Source: CAD feature listing. Evaluate the final solid. Frame: model axes, mm. A direction names the side the tool comes from. Give positions to 0.01 mm unless a question says otherwise; leave off trailing zeros. Order: outer loops, then holes, each group sorted by start corner. A loop starts at its lowest first (then second) coordinate and runs counter-clockwise, first axis right, second up.
from build123d import *

# Parameters (mm, degrees)
SALIENTE_EXTRUIR1_DEPTH = 6.35
CROQUIS2_R              = 6.35
CORTAR_EXTRUIR1_DEPTH   = 5
CROQUIS3_R              = 3.8
CORTAR_EXTRUIR2_DEPTH   = 2.35
CROQUIS6_R              = 1.5
CORTAR_EXTRUIR5_DEPTH   = 5
CROQUIS7_R              = 6.35
CORTAR_EXTRUIR6_DEPTH   = 5
CROQUIS8_R              = 3.5
CORTAR_EXTRUIR7_DEPTH   = 5
CROQUIS9_R              = 1.5
CORTAR_EXTRUIR8_DEPTH   = 5


with BuildPart() as part:
    # Croquis1 → Saliente-Extruir1 (new body)
    with BuildSketch(Plane.XY):
        with BuildLine():
            Line((10, 42.5), (10, -42.5))
            ThreePointArc((10, -42.5), (0, -52.5), (-10, -42.5))
            Line((-10, -42.5), (-10, 42.5))
            ThreePointArc((-10, 42.5), (0, 52.5), (10, 42.5))
        make_face()
    extrude(amount=SALIENTE_EXTRUIR1_DEPTH)

    # Croquis2 → Cortar-Extruir1 (cut)
    with BuildSketch(Plane.XY.offset(6.35)):
        with Locations((0, 42.5)):
            Circle(CROQUIS2_R)
    extrude(amount=-CORTAR_EXTRUIR1_DEPTH, mode=Mode.SUBTRACT)

    # Croquis3 → Cortar-Extruir2 (cut, through all)
    with BuildSketch(Plane.XY.offset(1.35)):
        with Locations((0, 42.5)):
            Circle(CROQUIS3_R)
    extrude(amount=-CORTAR_EXTRUIR2_DEPTH, mode=Mode.SUBTRACT)

    # Croquis6 → Cortar-Extruir5 (cut)
    with BuildSketch(Plane(origin=(10, 0, 0), x_dir=(0, 0, -1), z_dir=(1, 0, 0))):
        with Locations((-3.175, 42.5)):
            Circle(CROQUIS6_R)
    extrude(amount=-CORTAR_EXTRUIR5_DEPTH, mode=Mode.SUBTRACT)

    # Croquis7 → Cortar-Extruir6 (cut)
    with BuildSketch(Plane(origin=(0, 0, 0), x_dir=(-1, 0, 0), z_dir=(0, 0, -1))):
        with Locations((0, -42.5)):
            Circle(CROQUIS7_R)
    extrude(amount=-CORTAR_EXTRUIR6_DEPTH, mode=Mode.SUBTRACT)

    # Croquis8 → Cortar-Extruir7 (cut)
    with BuildSketch(Plane(origin=(0, 0, 5), x_dir=(-1, 0, 0), z_dir=(0, 0, -1))):
        with Locations((0, -42.5)):
            Circle(CROQUIS8_R)
    extrude(amount=-CORTAR_EXTRUIR7_DEPTH, mode=Mode.SUBTRACT)

    # Croquis9 → Cortar-Extruir8 (cut)
    with BuildSketch(Plane(origin=(10, 0, 0), x_dir=(0, 0, -1), z_dir=(1, 0, 0))):
        with Locations((-3.175, -42.5)):
            Circle(CROQUIS9_R)
    extrude(amount=-CORTAR_EXTRUIR8_DEPTH, mode=Mode.SUBTRACT)


solid = part.part
1) First-contact query: pin 1 Ø7 at (x, y) = (0, 42.5) entering from +Z; pin 2 Ø2.5 at (y, z) = (42.5, 3.175) entering from +X; pin 3 Ø1.5 at (x, z) = (-7.5, 1) entering from -Y. Flat tips, straight axial feed; report the tip coordinate or a pass-through.
Checks:
pin 1: passes through
pin 2: stops at x = -6.23
pin 3: stops at y = -49.88
2) Ray query, L1, parallel to Y at x = 0, z = 4.4; L2, parallel to Y at x = 0, z = 0.8; L3, parallel to X at y = -42.5, z = 1.5. Return the intervals inside material, ascending.
Checks:
L1: y = -52.5 to -48.85, -36.15 to 36.15, 48.85 to 52.5
L2: y = -52.5 to -48.85, -36.15 to 38.7, 46.3 to 52.5
L3: x = -10 to -6.35, 6.35 to 10
3) Section query A-A on x = 0. Output: boundary loops of the cut face in (y, z), and give its area (3 significant figures).
Checks:
outline: (-52.5, 0) - (-48.85, 0) - (-48.85, 5) - (-46, 5) - (-46, 6.35) - (-52.5, 6.35) - close; (-39, 5) - (-36.15, 5) - (-36.15, 0) - (38.7, 0) - (38.7, 1.35) - (36.15, 1.35) - (36.15, 6.35) - (-39, 6.35) - close; (46.3, 0) - (52.5, 0) - (52.5, 6.35) - (48.85, 6.35) - (48.85, 1.35) - (46.3, 1.35) - close
area: 520 mm2
4) Pull-direction query (X, two-part tool) for faces 6 (the face through (-10, -1, 3)), 7 (the face through (-0.2, 52.5, 3.1)), 8 (the face through (-3, -45, 5)); classes: +X half, -X half, draft (parallel to the pull), parting line (faces both ways), or undercut.
Checks:
face 6: -X half
face 7: parting line
face 8: undercut
5) Section query B-B on z = 3.75. Output: boundary loops of the cut face in (x, y).
Checks:
outline: (-10, -42.5) arc R10 ccw to (9.9, -43.89) - (6.2, -43.89) arc R6.35 cw (long way) to (6.2, -41.11) - (10, -41.11) - (10, 41.11) - (6.2, 41.11) arc R6.35 cw (long way) to (6.2, 43.89) - (9.9, 43.89) arc R10 ccw to (-10, 42.5) - close
6) Reachability of faces 1 (the face through (4, 43, 1.35)), 2 (the face through (0, 1, 6.35)), 3 (the face through (-6.057, -40.593, 2.465)), 4 (the face through (8.112, -43.964, 3.5)), 5 (the face through (0, 1, 0)) from +Z, -Z, +X, -X, +Y, -Y: full face, straight path, thin tool, end or side. Return the list, or none.
Checks:
face 1: +Z
face 2: +Z, +X, -X, +Y, -Y
face 3: -Z
face 4: +X
face 5: -Z, +X, -X, +Y, -Y
